Verification items for this drawing (mm, ordinates from the low corner). Round coordinates to 2 decimals unless told otherwise and drop trailing zeros. Order: outer loops, then holes, each group sorted by start corner. A loop starts at its lowest first (then second) coordinate and runs counter-clockwise, first axis right, second up. Notation, with made-up numbers: (32.25, 31) -> (71.25, 31) arc R28 ccw to (71.25, 54) -> close; hole circle Ø7 at (38, 37.5). An arc over 180 degrees is marked (long way). Return JSON: item names as keys, results as strings. Group by question number.
Item 1: Sectioned sample at B-B on y = 0.1. Record the cut outline in (x, z) (3 decimals), plus the area to 3 significant figures.
Item 2: Sectioned sample at A-A on x = 18. Record the cut outline in (y, z), plus the area to 3 significant figures.
Item 3: Scan lines: probe 1 along Z at (x, y) = (4.5, 0.2); probe 2 along X at (y, z) = (0.1, 0.6). Record each from-to range of solid material in increasing order. Write a range as from..to.
Item 4: Sectioned sample at C-C on z = 1.2. Record the cut outline in (x, y), plus the area to 3 significant figures.
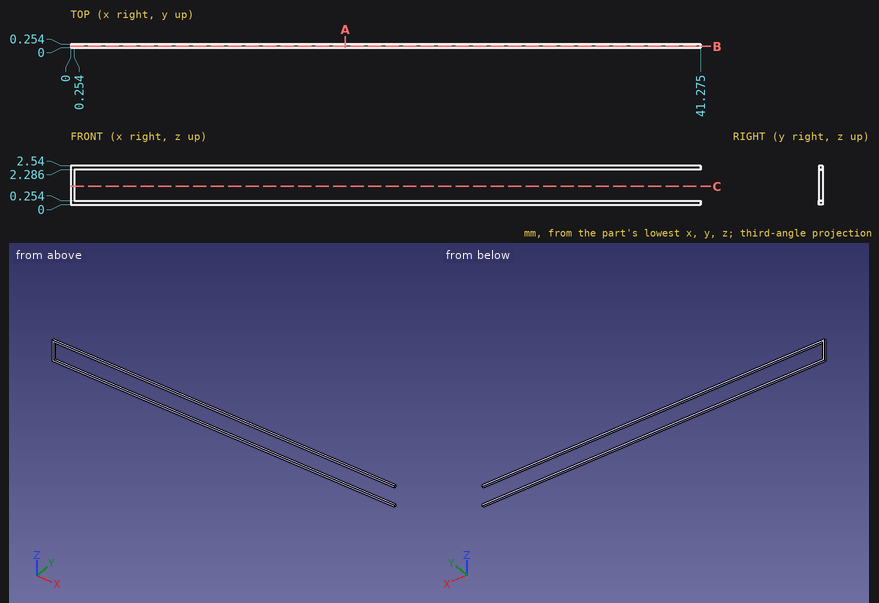
Recorded:
{
 "1": {"outline": "(0, 0) -> (41.275, 0) -> (41.275, 0.254) -> (0.254, 0.254) -> (0.254, 2.286) -> (41.275, 2.286) -> (41.275, 2.54) -> (0, 2.54) -> close", "area": "21.5 mm²"},
 "2": {"outline": "(0, 0) -> (0.25, 0) -> (0.25, 0.25) -> (0, 0.25) -> close; (0, 2.29) -> (0.25, 2.29) -> (0.25, 2.54) -> (0, 2.54) -> close", "area": "0.129 mm²"},
 "3": {"probe 1": "0..0.25, 2.29..2.54", "probe 2": "0..0.25"},
 "4": {"outline": "(0, 0) -> (0.25, 0) -> (0.25, 0.25) -> (0, 0.25) -> close", "area": "0.0645 mm²"}
}
